For this review, take the finished solid that the model builds, in its own axes (mm). A direction names the side the tool comes from. Coordinates: 2 decimals unless noted, no trailing zeros. Order: outer loops, then holes, each group sorted by start corner. A loop starts at its lowest first (then second) coordinate and runs counter-clockwise, first axis right, second up. Notation, with made-up numbers: (24.25, -15) -> (45.25, -15) arc R15 cw to (45.25, 0) -> close; hole circle Ø8 at (20, 68). An arc over 180 degrees is marked (long way). Return JSON: item names as keys, results as strings. Group by question number.
Item 1: Insertion check: pin 1 (1 mm diameter, centred on x = 19.5, y = 5.5, fed in from -Z); pin 2 (2 mm diameter, centred on x = 13.5, z = 14.5, fed in from -Y); pin 3 (1.2 mm diameter, centred on x = 8.5, y = 2, fed in from +Z). Each pin has a flat end and moves straight along its axis. Give the tip position at first contact, or say it passes through.
Item 2: Take a section at C-C (x = 17.5). Write out the cut boundary in (y, z).
Item 3: Take a section at A-A (z = 8.5). Write out the cut boundary in (x, y).
Item 4: Machinability: for faces 5 (the flat face through (6, 7, 4)), 6 (the flat face through (10.85, 10.14, 3.22)), 7 (the flat face through (1, 2.5, 14)), which of the approach directions +Z, -Z, +X, -X, +Y, -Y give a long, thin tool a straight path to every point of the face, cutting with its end or side? Answer none if there is none.
Item 5: Draft analysis for pull direction Y (two halves, no side actions). For faces 1 (the flat face through (6, 2.25, 8)), 2 (the flat face through (0, 10, 8)), 3 (the flat face through (6, 11.25, 9)), 4 (the flat face through (16, 2.5, 14)), state which applies: +Y half, -Y half, draft (parallel to the pull), parting line (faces both ways), or undercut.
Item 6: Take a section at D-D (z = 4.5). Write out the cut boundary in (x, y), then the cut area to 3 significant figures.
Item 7: For line 1 along X through (y, z) = (4, 12.5); line 2 along Y through (x, z) = (8.25, 8.25); line 3 along Y through (x, z) = (17.75, 13.5), list the stretches that pass through material, from the lowest coordinate up.
Item 8: Take a section at B-B (y = 4.5). Write out the cut boundary in (x, z).
```python
from build123d import *

# Parameters (mm, degrees)
BOX003_W               = 24
BOX003_H               = 23
BOX003_DEPTH           = 10
BOX003_ROLL_ANGLE      = -3.785379
BOX003_PITCH_ANGLE     = -4.658595
BOX003_PLACEMENT_ANGLE = 0.154031
BOX002_W               = 22
BOX002_H               = 2.5
BOX002_DEPTH           = 2.5
BOX001_W               = 9
BOX001_H               = 9
BOX001_DEPTH           = 11
BOX_W                  = 22
BOX_H                  = 20
BOX_DEPTH              = 15


with BuildPart() as cube003:
    # Box003 → Box003 (new body)
    with BuildSketch(Plane.XY):
        with Locations((12, 11.5)):
            Rectangle(BOX003_W, BOX003_H)
    extrude(amount=BOX003_DEPTH)


with BuildPart() as cube003_1:
    # Box003 roll: moved
    add(cube003.part.rotate(Axis((0, 0, 0), (1, 0, 0)), BOX003_ROLL_ANGLE))


with BuildPart() as cube003_2:
    # Box003 pitch: moved
    add(cube003_1.part.rotate(Axis((0, 0, 0), (0, 1, 0)), BOX003_PITCH_ANGLE))


with BuildPart() as cube003_3:
    # Box003 placement: moved
    add(cube003_2.part.moved(Location((-1, -2, -7))).rotate(Axis((-1, -2, -7), (0, 0, 1)), BOX003_PLACEMENT_ANGLE))


with BuildPart() as cube002:
    # Box002 → Box002 (new body)
    with BuildSketch(Plane.XY.offset(12.5)):
        with Locations((11, 1.25)):
            Rectangle(BOX002_W, BOX002_H)
    extrude(amount=BOX002_DEPTH)


with BuildPart() as cube001:
    # Box001 → Box001 (new body)
    with BuildSketch(Plane(origin=(1.25, 2.25, 4), x_dir=(1, 0, 0), z_dir=(0, 0, 1))):
        with Locations((4.5, 4.5)):
            Rectangle(BOX001_W, BOX001_H)
    extrude(amount=BOX001_DEPTH)


with BuildPart() as cut002:
    # Box → Box (new body)
    with BuildSketch(Plane.XY):
        with Locations((11, 10)):
            Rectangle(BOX_W, BOX_H)
    extrude(amount=BOX_DEPTH)

    # Cut: cut Cube001
    add(cube001.part, mode=Mode.SUBTRACT)

    # Cut001: cut Cube002
    add(cube002.part, mode=Mode.SUBTRACT)

    # Cut002: cut Cube003
    add(cube003_3.part, mode=Mode.SUBTRACT)


solid = cut002.part
```
Findings below:
{
 "1": {"pin 1": "stops at z = 4.18", "pin 2": "stops at y = 2.5", "pin 3": "stops at z = 12.5"},
 "2": {"outline": "(0, 4.43) -> (20, 3.11) -> (20, 15) -> (2.5, 15) -> (2.5, 12.5) -> (0, 12.5) -> close"},
 "3": {"outline": "(0, 0) -> (22, 0) -> (22, 20) -> (0, 20) -> close; hole (1.25, 2.25) -> (10.25, 2.25) -> (10.25, 11.25) -> (1.25, 11.25) -> close"},
 "4": {"face 5": "+Z", "face 6": "-Z, +X, -Y", "face 7": "+Z, +X, -X, -Y"},
 "5": {"face 1": "undercut", "face 2": "draft", "face 3": "undercut", "face 4": "-Y half"},
 "6": {"outline": "(0, 0) -> (18.31, 0) -> (22, 4.55) -> (22, 20) -> (0, 20) -> close; hole (1.25, 2.25) -> (10.25, 2.25) -> (10.25, 11.25) -> (1.25, 11.25) -> close", "area": "351 mm2"},
 "7": {"line 1": "x = 0 to 1.25, 10.25 to 22", "line 2": "y = 0 to 2.25, 11.25 to 20", "line 3": "y = 2.5 to 20"},
 "8": {"outline": "(0, 2.71) -> (22, 4.5) -> (22, 15) -> (10.25, 15) -> (10.25, 4) -> (1.25, 4) -> (1.25, 15) -> (0, 15) -> close"}
}
